Verification items for the finished model (mm, model axes). Face numbers are marked on the shaded views. A direction names the side the tool comes from. Coordinates: 2 decimals unless noted, no trailing zeros. Order: outer loops, then holes, each group sorted by start corner. A loop starts at its lowest first (then second) coordinate and runs counter-clockwise, first axis right, second up. Notation, with made-up numbers: M 19.25,0 L 26.25,0 A7 cw 26.25,8 Z; hole C 85.25,62 d7. An arc over 180 degrees is marked long. Return JSON: item names as keys, results as strings. Group by question number.
1. Gauge pin test, flat end, axial feed: pin 1 (4 mm diameter, centred on y = 23, z = 6.5, fed in from -X). Record the tip position at first contact, or that the pin passes through.
2. Section check D-D, the plane x = 17. Record the cut outline in (y, z), plus the area to 3 significant figures.
3. Section check C-C, the plane z = 7. Record the cut outline in (x, y), plus the area to 3 significant figures.
4. Mould release check, pull along X, two halves, no side actions. Record for the marked faces 1, 2 and 3: +X half, -X half, draft (parallel to the pull), parting line (faces both ways), or undercut.
5. Material ranges on line 1 along X through (y, z) = (12.5, 0.75) (3 decimals); line 2 along Z through (x, y) = (-22, 27) (3 decimals); line 3 along Z through (x, y) = (22, 21) (3 decimals), recorded low to high.
6. Section check B-B, the plane x = -18.5. Record the cut outline in (y, z).
7. Set-up check for the marked faces 4 and 5: record each of +Z, -Z, +X, -X, +Y, -Y from which the full face is reachable in a straight line by a thin tool's end or side.
8. Section check A-A, the plane y = 28. Record the cut outline in (x, z), plus the area to 3 significant figures.
Solid Edge part; units mm, degrees
sketch "Sketch1" plane through (0, 0, 0) normal (0, -1, 0) x (1, 0, 0)
  line L0 (10, 15) -> (-10, 15)
  line L1 (-10, -5) -> (-10, 15)
  line L2 (-10, -5) -> (-25, -5)
  line L3 (-25, -5) -> (-25, -15)
  line L4 (-25, -15) -> (25, -15)
  line L5 (25, -15) -> (25, -5)
  line L6 (10, -5) -> (25, -5)
  line L7 (10, -5) -> (10, 15)
extrude "Protrusion1" add sketch "Sketch1" against normal blind 40
sketch "Sketch2" plane through (25, 20, -10) normal (1, 0, 0) x (0, 1, 0)
  line L0 (20, 20) -> (-20, 5)
  line L1 (-20, 5) -> (20, 5)
  line L2 (20, 5) -> (20, 20)
extrude "ExtrudedProtrusion_3" add sketch "Sketch2" against normal blind 15
sketch "Sketch3" plane through (-25, 20, -10) normal (-1, 0, 0) x (0, -1, 0)
  line L0 (-20, 20) -> (20, 5)
  line L1 (20, 5) -> (-20, 5)
  line L2 (-20, 5) -> (-20, 20)
extrude "ExtrudedProtrusion_5" add sketch "Sketch3" against normal blind 15
sketch "Sketch4" plane through (0, 20, 15) normal (0, 0, 1) x (0, -1, 0)
  line L0 (-20, -20) -> (20, -10)
  line L1 (-20, -10) -> (-20, -20)
extrude "ExtrudedProtrusion_6" add sketch "Sketch4" against normal blind 20 material side at (-14.9515, 20.0121, 15)
sketch "Sketch5" plane through (0, 20, 15) normal (0, 0, 1) x (0, -1, 0)
  line L0 (-20, 20) -> (20, 10)
  line L1 (-20, 10) -> (-20, 20)
extrude "ExtrudedProtrusion_7" add sketch "Sketch5" against normal blind 20 material side at (14.9515, 20.0121, 15)
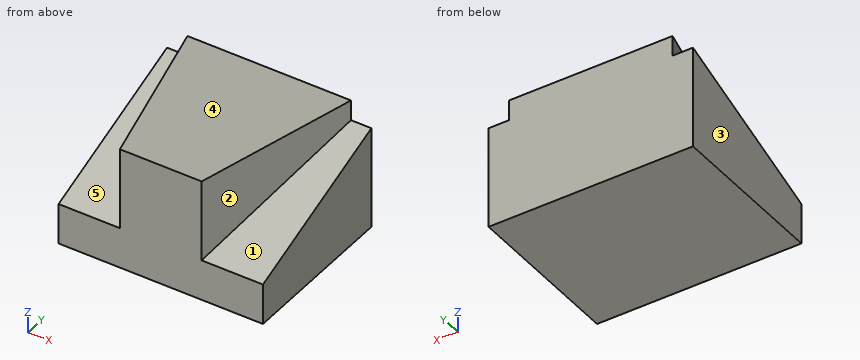
Answers follow:
{
 "1": {"pin 1": "x = -16.25"},
 "2": {"outline": "M 0,-15 L 40,-15 L 40,15 L 28,15 L 28,5.5 L 0,-5 Z", "area": "787 mm^2"},
 "3": {"outline": "M -25,32 L -18,32 L -10,0 L 10,0 L 18,32 L 25,32 L 25,40 L -25,40 Z", "area": "1,300 mm^2"},
 "4": {"face 1": "draft", "face 2": "+X half", "face 3": "-X half"},
 "5": {"line 1": "-13.125 to 13.125", "line 2": "-15 to 5.125", "line 3": "-15 to 2.875"},
 "6": {"outline": "M 0,-15 L 40,-15 L 40,15 L 34,15 L 34,7.75 L 0,-5 Z"},
 "7": {"face 4": "+Z, +X, -X, +Y, -Y", "face 5": "+Z, -X, -Y"},
 "8": {"outline": "M -25,-15 L 25,-15 L 25,5.5 L 17,5.5 L 17,15 L -17,15 L -17,5.5 L -25,5.5 Z", "area": "1,350 mm^2"}
}
